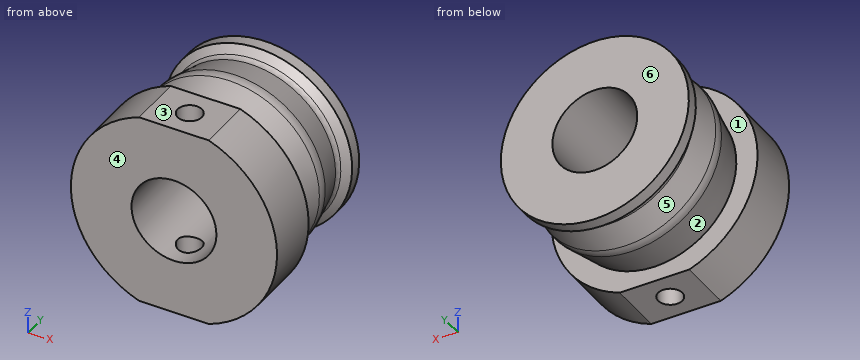
```python
from build123d import *

# Parameters (mm, degrees)
CUT_EXTRUDE1_DEPTH = 4.5
CHAMFER1_SIZE      = 1
CHAMFER1_SIZE_2    = 0.75
FILLET2_R          = 0.5


with BuildPart() as part:
    # Sketch2 → Revolve1 (revolve)
    with BuildSketch(Plane.XY, mode=Mode.PRIVATE) as revolve1_sk:
        with BuildLine():
            Line((3.5, 0), (3.5, 13))
            Line((3.5, 13), (7.75, 13))
            Line((7.75, 13), (7.75, 12))
            Line((7.75, 12), (6.75, 12))
            Line((6.75, 12), (7.456581804, 8.664472732))
            ThreePointArc((7.456581804, 8.664472732), (7.5, 8.25), (7.456581804, 7.835527268))
            Line((7.456581804, 7.835527268), (6.75, 4.5))
            Line((6.75, 4.5), (8.5, 4.5))
            Line((8.5, 4.5), (8.5, 0))
            Line((8.5, 0), (3.5, 0))
        make_face()
    revolve(revolve1_sk.sketch.rotate(Axis((0, 0, 0), (0, 1, 0)), 90), axis=Axis((0, 0, 0), (0, 1, 0)))

    # Sketch3 → Cut-Extrude1 (cut)
    with BuildSketch(Plane.XZ):
        with BuildLine():
            Line((-2.872281323, 8), (2.872281323, 8))
            ThreePointArc((2.872281323, 8), (0, 8.5), (-2.872281323, 8))
        make_face()
    cut_extrude1 = extrude(amount=-CUT_EXTRUDE1_DEPTH, mode=Mode.SUBTRACT)

    # Sketch5 → Ø2.0mm Dowel Hole1 (revolve, cut)
    with BuildSketch(Plane(origin=(0, 2.25, 8), x_dir=(0, -1, 0), z_dir=(1, 0, 0))):
        Polygon((0, 0), (0, 6.600860619), (1, 6), (1, 0), align=None)
    f_2_0mm_dowel_hole1 = revolve(axis=Axis((0, 2.25, 14.35), (0, 0, -1)), mode=Mode.SUBTRACT)

    # Mirror1: Cut-Extrude1, Ø2.0mm Dowel Hole1 across plane
    add(cut_extrude1.mirror(Plane.XY), mode=Mode.SUBTRACT)
    add(f_2_0mm_dowel_hole1.mirror(Plane.XY), mode=Mode.SUBTRACT)

    # Chamfer1
    # the kernel refuses this chamfer: 1, 0.75 mm, written as the material it adds along each edge
    with BuildSketch(Plane(origin=(0, 12, 0), x_dir=(0, 0, -1), z_dir=(1, 0, 0))) as chamfer1_piece_1:
        Polygon((6.75 + CHAMFER1_SIZE, 0), (6.75 + CHAMFER1_SIZE_2 * 0.20723636606, -CHAMFER1_SIZE_2 * 0.978290901819), (6.75, 0), align=None)
    revolve(axis=Axis((0, 12, 0), (0, 1, 0)))

    # Fillet2
    fillet2_edges = [part.edges().sort_by_distance(p)[0] for p in [
        (0, 11.266281824, 6.905427275),
    ]]
    fillet(fillet2_edges, radius=FILLET2_R)


solid = part.part
```
Input: part model. Units: mm. Frame: model coordinates. Face numbers are marked on the shaded views. A direction names the side the tool comes from. Give positions to 0.01 mm unless a question says otherwise; leave off trailing zeros. Order: outer loops, then holes, each group sorted by start corner. A loop starts at its lowest first (then second) coordinate and runs counter-clockwise, first axis right, second up.
1. Pin query (flat end, axial travel): pin 1 Ø2.5 at (x, y) = (0, 2.25) entering from -Z; pin 2 Ø5 at (x, y) = (-1, 10.5) entering from +Z; pin 3 Ø1 at (x, z) = (-2, 0) entering from -Y; pin 4 Ø1.5 at (y, z) = (9.5, -2.5) entering from +X. Return the tip coordinate at first contact, or that it passes through.
Computed:
pin 1: stops at z = -8
pin 2: stops at z = 7.75
pin 3: passes through
pin 4: stops at x = 7.13
2. Cut plane C-C (x = 0.25). State how many separate pieces and enclosed holes the cut face has, and give its area (3 significant figures).
Computed:
separate pieces: 4
enclosed holes: 0
area: 87.1 mm2
3. Cut plane B-B (y = 4.25). Return loops of the section in (x, z), and give its area (3 significant figures).
Computed:
outline: (-2.87, -8) - (2.87, -8) arc R8.5 ccw to (2.87, 8) - (-2.87, 8) arc R8.5 ccw to start; hole circle Ø7 at (0, 0)
area: 185 mm2
4. Set-up query: the marked faces 5 and 6. Return all of +Z, -Z, +X, -X, +Y, -Y with unobstructed straight access to the full face (end or side cutting, diameter ignored); none if empty.
Computed:
face 5: none
face 6: +Z, -Z, +X, -X, +Y
5. Draft query along Y for the marked faces 1, 2, 3 and 4. Return one class per face: released by +Y, released by -Y, zero draft, split by the parting line, or undercut.
Computed:
face 1: undercut
face 2: undercut
face 3: zero draft
face 4: released by -Y
6. Cut plane A-A (y = 2.25). Return loops of the section in (x, z).
Computed:
outline: (-2.87, -8) - (-1, -8) - (-1, -3.35) arc R3.5 cw to (-1, 3.35) - (-1, 8) - (-2.87, 8) arc R8.5 ccw to start; (1, -8) - (2.87, -8) arc R8.5 ccw to (2.87, 8) - (1, 8) - (1, 3.35) arc R3.5 cw to (1, -3.35) - close
7. Line query: probe 1 along Z at (x, y) = (4, 4); probe 2 along X at (y, z) = (2.25, -4.9); probe 3 along Y at (x, z) = (0, 5.1). Output: solid intervals per line, ascending.
Computed:
probe 1: z = -7.5 to 7.5
probe 2: x = -6.95 to -1, 1 to 6.95
probe 3: y = 0 to 1.25, 3.25 to 13
